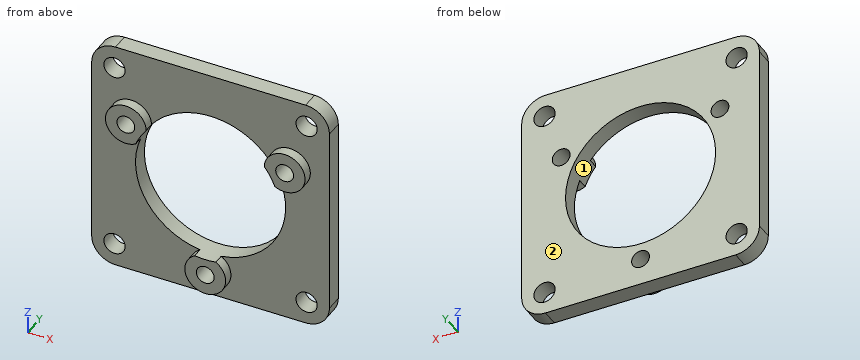
Autodesk Fusion 360 part; units mm, degrees
sketch "Sketch1" plane through (0, 0, 0) normal (0, 1, 0) x (1, 0, 0)
  line L0 (35, -35) -> (-35, -35)
  line L1 (-35, -35) -> (-35, 35)
  line L2 (-35, 35) -> (35, 35)
  line L3 (35, 35) -> (35, -35)
  line L4 (35, -35) -> (-35, 35) construction
  line L5 (-35, -35) -> (35, 35) construction
  dimension "d1" = 70
  dimension "d2" = 70
sketch "Sketch2" plane through (0, 0, 0) normal (0, 1, 0) x (1, 0, 0)
  line L0 (35, -35) -> (-35, 35)
  line L1 (28.2843, -28.2843) -> (-28.2843, -28.2843) construction
  line L2 (-28.2843, -28.2843) -> (-28.2843, 28.2843) construction
  line L3 (-28.2843, 28.2843) -> (28.2843, 28.2843) construction
  line L4 (28.2843, 28.2843) -> (28.2843, -28.2843) construction
  line L5 (28.2843, -28.2843) -> (-28.2843, 28.2843) construction
  line L6 (-28.2843, -28.2843) -> (28.2843, 28.2843) construction
  circle A0 centre (-28.2843, 28.2843) radius 3.125
  circle A1 centre (28.2843, 28.2843) radius 3.125
  circle A2 centre (-28.2843, -28.2843) radius 3.125
  circle A3 centre (28.2843, -28.2843) radius 3.125
  dimension "d6" = 80
  dimension "d7" = 6.25
  dimension "d12" = 6.25
  dimension "d13" = 6.25
  dimension "d14" = 6.25
sketch "Sketch3" plane through (0, 0, 0) normal (0, 1, 0) x (1, 0, 0)
  circle A0 centre (0, 0) radius 22.1
  dimension "d15" = 44.2
sketch "Sketch4" plane through (0, 0, 0) normal (0, 1, 0) x (1, 0, 0)
  circle A0 centre (0, 0) radius 27 construction
  circle A1 centre (0, 27) radius 2.625
  circle A2 centre (0, 27) radius 6
  circle A3 centre (-23.3827, -13.5) radius 2.625
  circle A4 centre (-23.3827, -13.5) radius 6
  circle A5 centre (23.3827, -13.5) radius 2.625
  circle A6 centre (23.3827, -13.5) radius 6
  dimension "d16" = 54
  dimension "d17" = 5.25
  dimension "d20" = 12
  dimension "d22" = 360
extrude "Extrude1" add sketch "Sketch1" against normal blind 5 makes body 1
extrude "Extrude4" add sketch "Sketch4" against normal blind 8 bodies 1
extrude "Extrude5" cut sketch "Sketch4" against normal up to surface (8 mm away) contours A1 | A3 | A5 bodies 1
fillet "Fillet1" radius 7 4 edges at (35, -2.5, 35) (35, -2.5, -35) (-35, -2.5, -35) (-35, -2.5, 35) on bodies 1
copy_body "Body->Comp1" bodies 1 removing the originals makes body 2 in component "Component"
extrude "Extrude1'" cut sketch "Sketch3" sketch "Sketch2" along normal up to surface of sketch 2 end surface through (0, -8, 0) normal (0, -1, 0) offset 0 bodies 2 in component "Component"
component "Component" placed x (1, 0, 0) y (0, 1, 0) z (0, 0, 1) at (0, 0, 0)
Can you work these out from the model? Positions are in its coordinate system, mm. Face numbers are marked on the shaded views. Coordinates: 2 decimals unless noted, no trailing zeros. Loops run counter-clockwise (first coordinate to the right, second up) from the corner with the lowest first, then second, coordinate; pieces in that order, holes last.
1) For pin 1 (8 mm diameter, centred on x = 28.28, z = -28.28, fed in from -Y); pin 2 (8 mm diameter, centred on x = 1, z = 25.5, fed in from +Y); pin 3 (1.5 mm diameter, centred on y = -6, z = -12, fed in from +X), each with a flat end and sliding along its axis, tell me the tip position at first contact or that it passes through.
2) Imagine slicing it at A-A on x = 0. List the corners of the cut face in (y, z) for me (3 decimals).
3) Imagine slicing it at C-C on x = -10.5. List the corners of the cut face in (y, z) for me.
4) Imagine slicing it at B-B on z = 0. List the corners of the cut face in (x, y) for me.
5) I need wall thicknesses on probe 1 along Z at (x, y) = (28.5, -3); probe 2 along Z at (x, y) = (0, -5.75) (3 decimals); probe 3 along X at (y, z) = (-2.5, 13.5). Which ranges of each line are inside material? Lowest first, please.
6) Thinking about a two-plate mould opening in X: for the marked faces 1 and 2, which applies, pulls with the +X half, pulls with the -X half, needs draft (parallel to the pull), parting line crosses it, or undercut?
7) Imagine slicing it at D-D on z = -27. List the corners of the cut face in (x, y) for me (3 decimals), plus the area to 3 significant figures.
Completed:
1. pin 1: stops at y = -5
1. pin 2: stops at y = 0
1. pin 3: passes through
2. outline: (-8, -33) - (-5, -33) - (-5, -35) - (0, -35) - (0, -29.625) - (-8, -29.625) - close; (-8, -24.375) - (0, -24.375) - (0, -22.1) - (-8, -22.1) - close; (-5, 22.1) - (0, 22.1) - (0, 35) - (-5, 35) - close
3. outline: (-5, -35) - (0, -35) - (0, -19.45) - (-5, -19.45) - close; (-5, 19.45) - (0, 19.45) - (0, 35) - (-5, 35) - close
4. outline: (-35, -5) - (-22.1, -5) - (-22.1, 0) - (-35, 0) - close; (22.1, -5) - (35, -5) - (35, 0) - (22.1, 0) - close
5. probe 1: z = -34.98 to -31.4, -25.17 to 25.17, 31.4 to 34.98
5. probe 2: z = -33 to -29.625, -24.375 to -22.1
5. probe 3: x = -35 to -26.01, -20.76 to -17.5, 17.5 to 20.76, 26.01 to 35
6. face 1: undercut
6. face 2: needs draft
7. outline: (-35, -5) - (-31.133, -5) - (-31.133, 0) - (-35, 0) - close; (-25.435, -5) - (-6, -5) - (-6, -8) - (-2.625, -8) - (-2.625, 0) - (-25.435, 0) - close; (2.625, -8) - (6, -8) - (6, -5) - (25.435, -5) - (25.435, 0) - (2.625, 0) - close; (31.133, -5) - (35, -5) - (35, 0) - (31.133, 0) - close
7. area: 287 mm2
